```python
from build123d import *

# Parameters (mm, degrees)
SKETCH_1_W          = 20
SKETCH_1_H          = 50
EXTRUDE_1_DEPTH     = 3
SKETCH_2_R          = 7.5
EXTRUDE_2_DEPTH     = 5
SKETCH_3_R          = 3
CUT_EXTRUDE_1_DEPTH = 2.5
SKETCH_4_R          = 2.5
CUT_EXTRUDE_2_DEPTH = 3


with BuildPart() as part:
    # 草图1 → 凸台-拉伸1 (new body)
    with BuildSketch(Plane.XY):
        Rectangle(SKETCH_1_W, SKETCH_1_H)
    extrude(amount=EXTRUDE_1_DEPTH)

    # 草图2 → 凸台-拉伸2 (add)
    with BuildSketch(Plane.XY.offset(3)):
        Circle(SKETCH_2_R)
    extrude(amount=EXTRUDE_2_DEPTH)

    # 草图3 → 切除-拉伸1 (cut)
    with BuildSketch(Plane.XY.offset(8)):
        Circle(SKETCH_3_R)
    extrude(amount=-CUT_EXTRUDE_1_DEPTH, mode=Mode.SUBTRACT)

    # 草图4 → 切除-拉伸2 (cut)
    with BuildSketch(Plane.XY.offset(3)):
        with Locations((0, 18)):
            Circle(SKETCH_4_R)
        with Locations((-0.580661347, -18)):
            Circle(SKETCH_4_R)
    extrude(amount=-CUT_EXTRUDE_2_DEPTH, mode=Mode.SUBTRACT)


solid = part.part
```
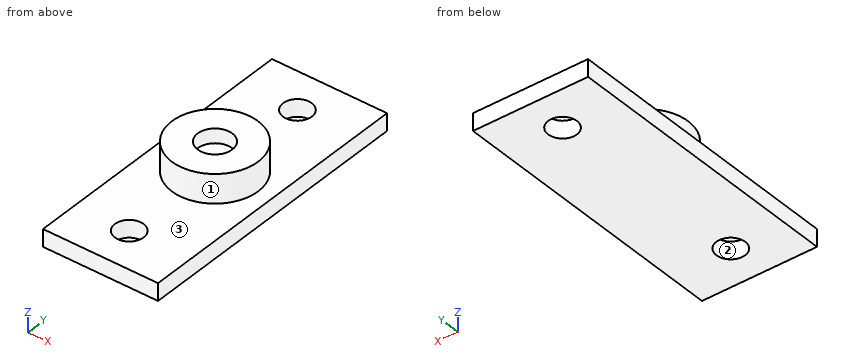
Can you work these out from the model? Positions are in its coordinate system, mm. Face numbers are marked on the shaded views. Coordinates: 2 decimals unless noted, no trailing zeros. Loops run counter-clockwise (first coordinate to the right, second up) from the corner with the lowest first, then second, coordinate; pieces in that order, holes last. Notation, with made-up numbers: (-30, -7.5) - (-19, -7.5) arc R32 cw to (-19, 27.5) - close; hole circle Ø7 at (-30.75, 9.25). An arc over 180 degrees is marked (long way). Answer as CSV lines item,"result". Start each with the question number.
1) Suppose I cut it at A-A (y = -18). Please give me the cut outline in (x, z), plus the area to 3 significant figures.
2) I need wall thicknesses on line 1 (Y direction, x = 1, z = 1.25); line 2 (Y direction, x = 0, z = 6.1); line 3 (Z direction, x = 4, y = 17.5). Which ranges of each line are inside material? Lowest first, please. Write a range as from..to.
3) Suppose I cut it at C-C (x = 0). Please give me the cut outline in (y, z), plus the area to 3 significant figures.
4) Suppose I cut it at D-D (x = 4). Please give me the cut outline in (y, z).
5) Suppose I cut it at B-B (z = 2). Please give me the cut outline in (x, y).
6) Thinking about a two-plate mould opening in X: for the marked faces 1, 2 and 3, which applies, pulls with the +X half, pulls with the -X half, needs draft (parallel to the pull), parting line crosses it, or undercut?
7) For pin 1 (2 mm diameter, centred on x = -3.5, z = 5.5, fed in from -Y); pin 2 (1 mm diameter, centred on x = -2, y = 11.5, fed in from +Z); pin 3 (3 mm diameter, centred on x = -0.5, y = -1, fed in from +Z), each with a flat end and sliding along its axis, tell me the tip position at first contact or that it passes through.
Check result:
1,outline,"(-10, 0) - (-3.08, 0) - (-3.08, 3) - (-10, 3) - close; (1.92, 0) - (10, 0) - (10, 3) - (1.92, 3) - close"
1,area,"45.0 mm²"
2,line 1,"y = -25..-19.94, -16.06..15.71, 20.29..25"
2,line 2,"y = -7.5..-3, 3..7.5"
2,line 3,"z = 0..3"
3,outline,"(-25, 0) - (-20.43, 0) - (-20.43, 3) - (-25, 3) - close; (-15.57, 0) - (15.5, 0) - (15.5, 3) - (7.5, 3) - (7.5, 8) - (3, 8) - (3, 5.5) - (-3, 5.5) - (-3, 8) - (-7.5, 8) - (-7.5, 3) - (-15.57, 3) - close; (20.5, 0) - (25, 0) - (25, 3) - (20.5, 3) - close"
3,area,"180 mm²"
4,outline,"(-25, 0) - (25, 0) - (25, 3) - (6.34, 3) - (6.34, 8) - (-6.34, 8) - (-6.34, 3) - (-25, 3) - close"
5,outline,"(-10, -25) - (10, -25) - (10, 25) - (-10, 25) - close; hole circle Ø5 at (-0.58, -18); hole circle Ø5 at (0, 18)"
6,face 1,"parting line crosses it"
6,face 2,"undercut"
6,face 3,"needs draft"
7,pin 1,"stops at y = -7.07"
7,pin 2,"stops at z = 3"
7,pin 3,"stops at z = 5.5"
